from build123d import *

# Parameters (mm, degrees)
BOSS_EXTRUDE1_DEPTH = 1.8
SKETCH2_R           = 1.5
CUT_EXTRUDE2_DEPTH  = 1.8


with BuildPart() as part:
    # Sketch1 → Boss-Extrude1 (new body)
    with BuildSketch(Plane(origin=(0, 0, 0), x_dir=(1, 0, 0), z_dir=(0, 1, 0))):
        Polygon((0, 0), (60, 0), (99.244426356, -39.244426356), (99.244426356, -54.244426356), (81.244426356, -54.244426356), (47.5, -21.528777349), (12.5, -21.528777349), (-21.244426356, -54.244426356), (-39.244426356, -54.244426356), (-39.244426356, -39.244426356), align=None)
    extrude(amount=BOSS_EXTRUDE1_DEPTH)

    # Sketch2 → Cut-Extrude2 (cut)
    with BuildSketch(Plane(origin=(0, 1.8, 0), x_dir=(1, 0, 0), z_dir=(0, 1, 0))):
        with Locations(Location((-4.75, -13, 0), (0, 0, 270))):
            Circle(SKETCH2_R)
        with Locations(Location((64.75, -13, 0), (0, 0, 270))):
            Circle(SKETCH2_R)
    extrude(amount=-CUT_EXTRUDE2_DEPTH, mode=Mode.SUBTRACT)


solid = part.part
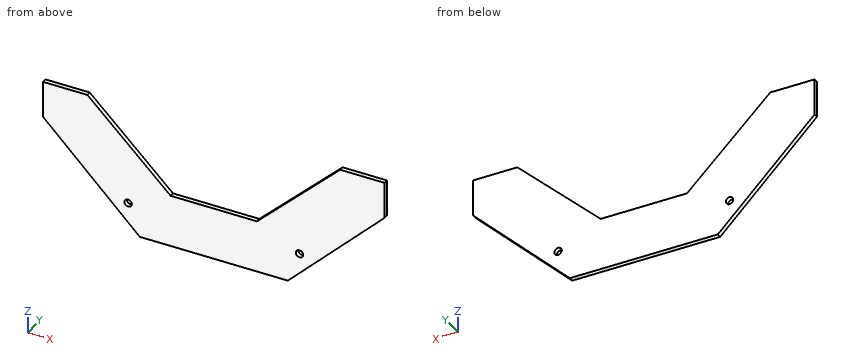
Design review of the part built by this model. Coordinates are the model's own, in mm. Coordinates: 2 decimals unless noted, no trailing zeros. Loops run counter-clockwise (first coordinate to the right, second up) from the corner with the lowest first, then second, coordinate; pieces in that order, holes last. Notation, with made-up numbers: M 8.25,-3 L 19.25,-3 A28 ccw 19.25,26 Z; hole C 51,49 d8. An arc over 180 degrees is marked long. Answer as CSV lines item,"result".
Item 1: Add section D-D on z = 41.5. State the section outline as (x, y) points.
Answer list:
outline,"M -39.24,0 L -8.1,0 L -8.1,1.8 L -39.24,1.8 Z; M 68.1,0 L 99.24,0 L 99.24,1.8 L 68.1,1.8 Z"
Item 2: Add section A-A on z = 13. State the section outline as (x, y) points.
Answer list:
outline,"M -13,0 L -6.25,0 L -6.25,1.8 L -13,1.8 Z; M -3.25,0 L 63.25,0 L 63.25,1.8 L -3.25,1.8 Z; M 66.25,0 L 73,0 L 73,1.8 L 66.25,1.8 Z"
Item 3: Add section B-B on x = 64.75. State the section outline as (y, z) points.
Answer list:
outline,"M 0,4.75 L 1.8,4.75 L 1.8,11.5 L 0,11.5 Z; M 0,14.5 L 1.8,14.5 L 1.8,38.25 L 0,38.25 Z"
Item 4: For probe 1 along X at (y, z) = (1.3, 13); probe 2 along X at (y, z) = (1.2, 12.5); probe 3 along X at (y, z) = (0.65, 22), list the stretches that pass through material, from the lowest coordinate up.
Answer list:
probe 1,"-13 to -6.25, -3.25 to 63.25, 66.25 to 73"
probe 2,"-12.5 to -6.16, -3.34 to 63.34, 66.16 to 72.5"
probe 3,"-22 to 12.01, 47.99 to 82"
Item 5: Add section C-C on y = 0.9. State the section outline as (x, z) points.
Answer list:
outline,"M -39.24,39.24 L 0,0 L 60,0 L 99.24,39.24 L 99.24,54.24 L 81.24,54.24 L 47.5,21.53 L 12.5,21.53 L -21.24,54.24 L -39.24,54.24 Z; hole C -4.75,13 d3; hole C 64.75,13 d3"
